```python
from build123d import *

# Parameters (mm, degrees)
BOSS_EXTRUDE1_DEPTH = 1825
DOWN_DEPTH          = 47
UP_DEPTH            = 75


with BuildPart() as part:
    # Sketch1 → Boss-Extrude1 (new body)
    with BuildSketch(Plane.XY):
        Polygon((0, 0), (0, 20), (50, 20), (50, 0), (47, 0), (47, 17), (3, 17), (3, 0), align=None)
    extrude(amount=BOSS_EXTRUDE1_DEPTH)

    # Sketch2 → Down (add)
    with BuildSketch(Plane.XY.offset(1825)):
        Polygon((0, 0), (0, 20), (50, 20), (50, 0), (47, 0), (47, 17), (3, 17), (3, 0), align=None)
    extrude(amount=DOWN_DEPTH)

    # Sketch3 → Up (add)
    with BuildSketch(Plane(origin=(0, 0, 0), x_dir=(-1, 0, 0), z_dir=(0, 0, -1))):
        Polygon((-50, 0), (-50, 20), (0, 20), (0, 0), (-3, 0), (-3, 17), (-47, 17), (-47, 0), align=None)
    extrude(amount=UP_DEPTH)


solid = part.part
```
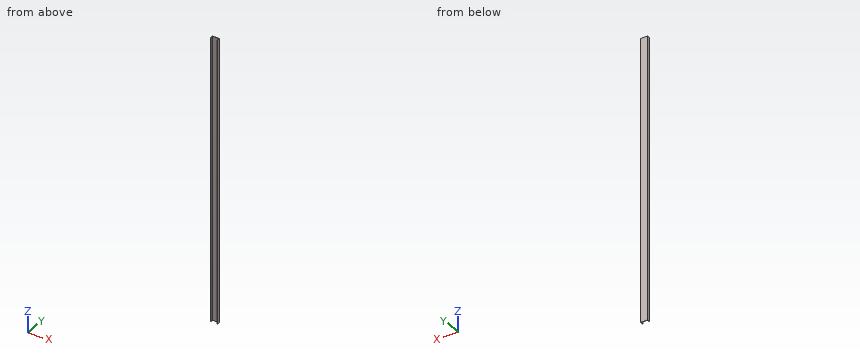
Input: part model. Units: mm. Frame: model coordinates. Coordinates: 2 decimals unless noted, no trailing zeros. Loops run counter-clockwise (first coordinate to the right, second up) from the corner with the lowest first, then second, coordinate; pieces in that order, holes last.
Q1. Line query: line 1 along X through (y, z) = (14.5, 1243); line 2 along Y through (x, z) = (35.5, 1203). Output: solid intervals per line, ascending.
Results are:
line 1: x = 0 to 3, 47 to 50
line 2: y = 17 to 20
Q2. Section A-A, the plane y = 4.75. Return the cut outline in (x, z), and give its area (3 significant figures).
Results are:
outline: (0, -75) - (3, -75) - (3, 1872) - (0, 1872) - close; (47, -75) - (50, -75) - (50, 1872) - (47, 1872) - close
area: 11,700 mm2
Q3. Contact query for a flat-ended pin moving along its axis: pin 1 (22 mm diameter, centred on x = 16, z = 1114.5, fed in from -Y). Output: stop coordinate, or through.
Results are:
pin 1: stops at y = 17
Q4. Section B-B, the plane z = 1202. Return the cut outline in (x, y).
Results are:
outline: (0, 0) - (3, 0) - (3, 17) - (47, 17) - (47, 0) - (50, 0) - (50, 20) - (0, 20) - close
Q5. Section C-C, the plane x = 24.5. Return the cut outline in (y, z), and give its area (3 significant figures).
Results are:
outline: (17, -75) - (20, -75) - (20, 1872) - (17, 1872) - close
area: 5,840 mm2
